Can you work these out from the drawing? Everything is in mm from the part's minimum corner. Round coordinates to 2 decimals unless told otherwise and drop trailing zeros. Loops run counter-clockwise (first coordinate to the right, second up) from the corner with the lowest first, then second, coordinate; pieces in that order, holes last. Notation, with made-up numbers: (61.5, 9) -> (82.5, 9) arc R29 ccw to (82.5, 42) -> close; hole circle Ø9 at (-15, -8). An arc over 180 degrees is marked (long way). Answer as a JSON object with one key per item and string values.
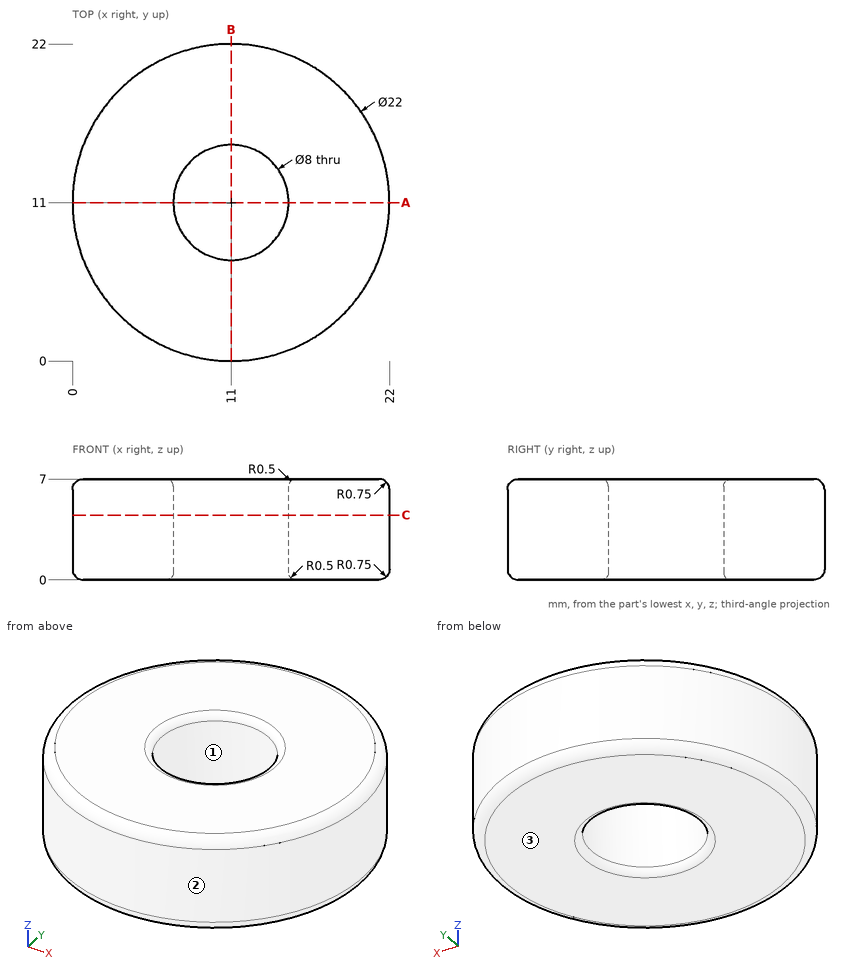
Q1. I'm going to push flat-ended pins straight in: pin 1 (1 mm diameter, centred on y = 4.5, z = 4, fed in from -X); pin 2 (4 mm diameter, centred on y = 15.5, z = 5, fed in from +X); pin 3 (1.5 mm diameter, centred on x = 7.5, z = 1.5, fed in from -Y). Where does each tip first touch, or does it pass through?
Determined:
{"pin 1": "x = 1.78", "pin 2": "x = 21.71", "pin 3": "y = 0.35"}
Q2. If I drill on L1, parallel to Y at x = 11, z = 1.75; L2, parallel to Y at x = 12, z = 4.5; L3, parallel to X at y = 12.5, z = 0.5, over which ranges is the centre line in solid material (lowest first)? Write a range as [from, to].
Determined:
{"L1": "[0, 7], [15, 22]", "L2": "[0.05, 7.13], [14.87, 21.95]", "L3": "[0.15, 7.29], [14.71, 21.85]"}
Q3. We'd pull the mould along X, two halves only. Please class the marked faces 1, 2 and 3: pulls with the +X half, pulls with the -X half, needs draft (parallel to the pull), parting line crosses it, or undercut.
Determined:
{"face 1": "undercut", "face 2": "parting line crosses it", "face 3": "needs draft"}
Q4. I want a section at C-C, the plane z = 4.5. Write out the boundary of the cut face in (x, y).
Determined:
{"outline": "circle Ø22 at (11, 11); hole circle Ø8 at (11, 11)"}
Q5. I want a section at A-A, the plane y = 11. Write out the boundary of the cut face in (x, z), then the cut area to 3 significant figures.
Determined:
{"outline": "(0, 0.75) arc R0.75 ccw to (0.75, 0) -> (6.5, 0) arc R0.5 ccw to (7, 0.5) -> (7, 6.5) arc R0.5 ccw to (6.5, 7) -> (0.75, 7) arc R0.75 ccw to (0, 6.25) -> close; (15, 0.5) arc R0.5 ccw to (15.5, 0) -> (21.25, 0) arc R0.75 ccw to (22, 0.75) -> (22, 6.25) arc R0.75 ccw to (21.25, 7) -> (15.5, 7) arc R0.5 ccw to (15, 6.5) -> close", "area": "97.3 mm²"}
